Geometry: final body of the model. Coordinates: model frame, mm. A direction names the side the tool comes from. Coordinates: 2 decimals unless noted, no trailing zeros. Write item = value, one per line. Start each with the question number.
Item 1: Pull-direction query (Z, two-part tool) for faces 1 (the cylindrical face through (141.66, 13.11, 43.8)), 2 (the flat face through (57.857, 31, 60)), 3 (the cylindrical face through (134.7, 3.5, 9)); classes: +Z half, -Z half, draft (parallel to the pull), parting line (faces both ways), or undercut.
Item 2: First-contact query: pin 1 Ø4.5 at (y, z) = (33, 36.5) entering from +X; pin 2 Ø10 at (x, y) = (99.5, 31.5) entering from +Z; pin 3 Ø10 at (x, y) = (15, 44) entering from +Z. Flat tips, straight axial feed; report the tip coordinate or a pass-through.
Item 3: Ray query, L1, parallel to X at y = 11, z = 127; L2, parallel to Z at x = 35, y = 27; L3, parallel to Z at x = 139, y = 52. Return the intervals inside material, ascending. Write a range as [from, to].
Item 4: Reachability of faces 4 (the cylindrical face through (140.62, 21, 37.27)), 5 (the cylindrical face through (2.82, 21, 134.97)), 6 (the flat face through (123, 7, 25)) from +Z, -Z, +X, -X, +Y, -Y: full face, straight path, thin tool, end or side. Return the list, or none.
Item 5: Section A-A on y = 28. Give the number of separate pieces and of enclosed holes in the cut face, plus the area to 3 significant figures.
from build123d import *

# Parameters (mm, degrees)
BOSS_EXTRUDE1_DEPTH = 1000
SKETCH2_R           = 3
CUT_EXTRUDE2_DEPTH  = 1016.012315196
SKETCH3_R           = 30
CUT_EXTRUDE3_DEPTH  = 67


with BuildPart() as part:
    # Sketch1 → Boss-Extrude1 (new body)
    with BuildSketch(Plane.XY):
        Polygon((11.571428571, 55), (11.571428571, 7), (3, 7), (3, 55), (0, 55), (0, 7), (0, 0), (165, 0), (165, 7), (165, 10), (165, 55), (162, 55), (162, 7), (153.428571429, 7), (153.428571429, 55), (150.428571429, 55), (150.428571429, 7), (141.857142857, 7), (141.857142857, 55), (138.857142857, 55), (138.857142857, 7), (130.285714286, 7), (130.285714286, 55), (127.285714286, 55), (127.285714286, 7), (118.714285714, 7), (118.714285714, 55), (115.714285714, 55), (115.714285714, 7), (107.142857143, 7), (107.142857143, 55), (104.142857143, 55), (104.142857143, 7), (95.571428571, 7), (95.571428571, 55), (92.571428571, 55), (92.571428571, 7), (84, 7), (84, 55), (81, 55), (81, 7), (72.428571429, 7), (72.428571429, 55), (69.428571429, 55), (69.428571429, 7), (60.857142857, 7), (60.857142857, 55), (57.857142857, 55), (57.857142857, 7), (49.285714286, 7), (49.285714286, 55), (46.285714286, 55), (46.285714286, 7), (37.714285714, 7), (37.714285714, 55), (34.714285714, 55), (34.714285714, 7), (26.142857143, 7), (26.142857143, 55), (23.142857143, 55), (23.142857143, 7), (14.571428571, 7), (14.571428571, 55), align=None)
    extrude(amount=BOSS_EXTRUDE1_DEPTH)

    # Sketch2 → Cut-Extrude2 (cut, through all)
    with BuildSketch(Plane.XZ):
        with BuildLine():
            Line((0, 1000), (0, 135))
            ThreePointArc((0, 135), (8.829422446, 134.710954637), (17.62103595, 133.845056285))
            Line((17.62103595, 133.845056285), (32.26946717, 144.181033328))
            ThreePointArc((32.26946717, 144.181033328), (38.952266288, 145.371836857), (44.144338328, 140.999171191))
            Line((44.144338328, 140.999171191), (51.662263369, 124.723736889))
            ThreePointArc((51.662263369, 124.723736889), (67.5, 116.913429511), (82.182792916, 107.102700939))
            Line((82.182792916, 107.102700939), (101.156071179, 110.411535956))
            ThreePointArc((101.156071179, 110.411535956), (108.187337522, 108.187337522), (110.411535956, 101.156071179))
            Line((110.411535956, 101.156071179), (107.102700939, 82.182792916))
            ThreePointArc((107.102700939, 82.182792916), (116.913429511, 67.5), (124.723736889, 51.662263369))
            Line((124.723736889, 51.662263369), (140.999171191, 44.144338328))
            ThreePointArc((140.999171191, 44.144338328), (145.371836857, 38.952266288), (144.181033328, 32.26946717))
            Line((144.181033328, 32.26946717), (133.845056285, 17.62103595))
            ThreePointArc((133.845056285, 17.62103595), (134.710954637, 8.829422446), (135, 0))
            Line((135, 0), (165, 0))
            Line((165, 0), (165, 1000))
            Line((165, 1000), (0, 1000))
        make_face()
        with Locations(Location((36.881713927, 137.644430246, 0), (0, 0, 270))):
            Circle(SKETCH2_R)
        with Locations(Location((102.530483272, 102.530483272, 0), (0, 0, 270))):
            Circle(SKETCH2_R)
        with Locations(Location((137.644430246, 36.881713927, 0), (0, 0, 270))):
            Circle(SKETCH2_R)
    extrude(amount=-CUT_EXTRUDE2_DEPTH, mode=Mode.SUBTRACT)

    # Sketch3 → Cut-Extrude3 (cut)
    with BuildSketch(Plane(origin=(0, 55, 0), x_dir=(1, 0, 0), z_dir=(0, 1, 0))):
        Circle(SKETCH3_R)
    extrude(amount=-CUT_EXTRUDE3_DEPTH, mode=Mode.SUBTRACT)


solid = part.part
Responses:
q1.face_1 = parting line
q1.face_2 = draft
q1.face_3 = undercut
q2.pin_1 = 141.86
q2.pin_2 = 110.37
q2.pin_3 = 134.5
q3.L1 = [0, 3], [11.57, 14.57], [23.14, 26.14], [34.71, 37.71], [46.29, 49.29]
q3.L2 = [0, 135.31], [139.98, 145.42]
q3.L3 = [24.93, 34.21], [39.56, 45.07]
q4.face_4 = +Y, -Y
q4.face_5 = +Z, +Y, -Y
q4.face_6 = +Z, -Z, +Y
q5.separate_pieces = 14
q5.enclosed_holes = 0
q5.area = 3,900 mm²
